The model under review builds one solid part; all positions refer to its coordinate system, in mm. A direction names the side the tool comes from. Round coordinates to 2 decimals unless told otherwise and drop trailing zeros. Write each loop counter-clockwise with the first axis right and the second up, starting at its lowest first coordinate (ties: lowest second). Pieces come first, ordered by that corner, then holes. Notation, with made-up numbers: M 6.25,13.25 L 42.25,13.25 A33 ccw 42.25,43.25 Z; hole C 45.25,21 d5. An arc over 180 degrees is marked long. Write item = value, one per line. Start each with the question number.
Item 1: Take a section at D-D, the plane z = -4. Give the boundary of the cut face in (x, y).
Item 2: Tool access review of faces 1 (the flat face through (2, 0, 0)), 2 (the flat face through (0.2, 4, 1)): name each direction out of +Z, -Z, +X, -X, +Y, -Y from which nothing blocks a thin tool from reaching the whole face with its end or side.
Item 3: To check wall thickness, follow line 1 along Y through (x, z) = (0.1, 0); line 2 along Y through (x, z) = (0.3, 0); line 3 along X through (y, z) = (-0.25, -1.5). State the ranges of each line that lie inside material, in increasing order.
Item 4: The part is to be moulded in two halves that separate along Y. For faces 3 (the cylindrical face through (0.99, -4.88, 1.08)), 4 (the flat face through (0.2, 0.5, 0)), 5 (the flat face through (0, -2, 2)), say which applies: +Y half, -Y half, draft (parallel to the pull), parting line (faces both ways), or undercut.
Item 5: Take a section at A-A, the plane z = 0. Give the boundary of the cut face in (x, y).
Item 6: Take a section at C-C, the plane x = 1.4. Give the boundary of the cut face in (y, z), plus the area to 3 significant figures.
from build123d import *

# Parameters (mm, degrees)
SKETCH_1_R          = 5
EXTRUDE_310_DEPTH   = 2
SKETCH_9_R          = 4.442422665
CUT_EXTRUDE_1_DEPTH = 0.2
SKETCH_10_R         = 3.682968426
EXTRUDE_1_DEPTH     = 0.2
SKETCH_11_R         = 2.01865338
CUT_EXTRUDE_2_DEPTH = 0.2
SKETCH_12_R         = 0.285545309
CUT_EXTRUDE_3_DEPTH = 0.4


with BuildPart() as part:
    # 草图1 → Extrude 310 (new body)
    with BuildSketch(Plane(origin=(0, 0, 0), x_dir=(0, 0, -1), z_dir=(1, 0, 0))):
        Circle(SKETCH_1_R)
    extrude(amount=EXTRUDE_310_DEPTH)

    # 草图9 → 切除-拉伸1 (cut)
    with BuildSketch(Plane.ZY):
        Circle(SKETCH_9_R)
    extrude(amount=-CUT_EXTRUDE_1_DEPTH, mode=Mode.SUBTRACT)

    # 草图10 → 凸台-拉伸1 (add)
    with BuildSketch(Plane.ZY.offset(-0.2)):
        Circle(SKETCH_10_R)
    extrude(amount=EXTRUDE_1_DEPTH)

    # 草图11 → 切除-拉伸2 (cut)
    with BuildSketch(Plane.ZY):
        Circle(SKETCH_11_R)
    extrude(amount=-CUT_EXTRUDE_2_DEPTH, mode=Mode.SUBTRACT)

    # 草图12 → 切除-拉伸3 (cut)
    with BuildSketch(Plane.ZY.offset(-0.2)):
        Circle(SKETCH_12_R)
    extrude(amount=-CUT_EXTRUDE_3_DEPTH, mode=Mode.SUBTRACT)


solid = part.part
Response values:
q1.outline = M 0,-3 L 2,-3 L 2,3 L 0,3 L 0,1.93 L 0.2,1.93 L 0.2,-1.93 L 0,-1.93 Z
q2.face_1 = +Z, -Z, +X, +Y, -Y
q2.face_2 = -X
q3.line_1 = -5 to -4.44, -3.68 to -2.02, 2.02 to 3.68, 4.44 to 5
q3.line_2 = -5 to -0.29, 0.29 to 5
q3.line_3 = 0.2 to 2
q4.face_3 = parting line
q4.face_4 = undercut
q4.face_5 = draft
q5.outline = M 0,-5 L 2,-5 L 2,5 L 0,5 L 0,4.44 L 0.2,4.44 L 0.2,3.68 L 0,3.68 L 0,2.02 L 0.2,2.02 L 0.2,0.29 L 0.6,0.29 L 0.6,-0.29 L 0.2,-0.29 L 0.2,-2.02 L 0,-2.02 L 0,-3.68 L 0.2,-3.68 L 0.2,-4.44 L 0,-4.44 Z
q6.outline = C 0,0 d10
q6.area = 78.5 mm2
